Build history of the part. All positions in model axes, mm. Face numbers are marked on the shaded views. A direction names the side the tool comes from. Give positions to 0.01 mm unless a question says otherwise; leave off trailing zeros. Order: outer loops, then holes, each group sorted by start corner. A loop starts at its lowest first (then second) coordinate and runs counter-clockwise, first axis right, second up. Notation, with made-up numbers: (53, -28) - (76, -28) arc R14 cw to (76, -2) - close; hole circle Ø11 at (23.25, -38.75). An arc over 180 degrees is marked (long way). Use a Markdown table: item, result. Add a question column.
(1) Flat gauge pins, fed straight in: pin 1 (4 mm diameter, centred on x = 1.5, z = 11.5, fed in from -Y); pin 2 (6 mm diameter, centred on y = -23.5, z = 13.5, fed in from +X); pin 3 (2.5 mm diameter, centred on x = 68, z = 13, fed in from -Y). Where does each tip first touch, or does it go through?
(2) Slice it at B-B (z = 7.75). Write the cut outline in (x, y), then the cut area to 3 significant figures.
(3) Slice it at A-A (y = -28.5). Write the cut outline in (x, z), then the cut area to 3 significant figures.
(4) Wall check: line 1 (X direction, y = -19.5, z = 16.5); line 2 (X direction, y = -33, z = 14.5); line 3 (Y direction, x = 62, z = 2). Give the ranges that are in metal, low to high.
(5) Which spindle directions (+Z, -Z, +X, -X, +Y, -Y) get a long thin tool onto all of the face, cutting with end or side? Do the marked faces 1, 2 and 3. Say none if no direction does.
(6) Mould opens along X. For the marked faces 4, 5, 6 and 7 say: +X half, -X half, draft (parallel to the pull), parting line (faces both ways), or undercut.
(7) Slice it at C-C (x = 68). Write the cut outline in (y, z).
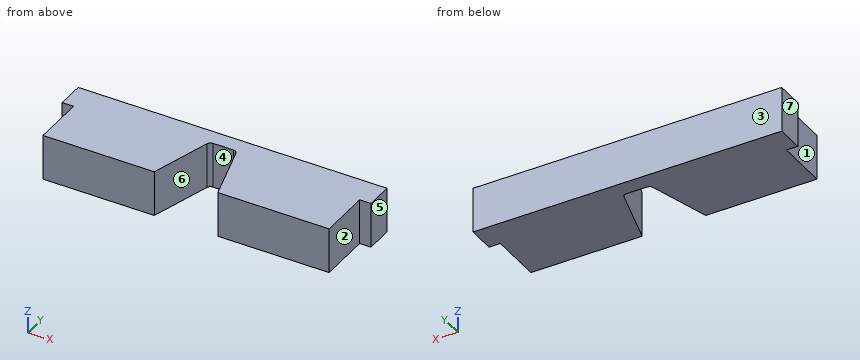
from build123d import *

# Parameters (mm, degrees)
F0_W     = 136
F0_H     = 35
F1_DEPTH = 20
F2_W     = 5
F2_H     = 23
F3_DEPTH = 25
F4_R     = 2


with BuildPart() as f1:
    # F0 (on Top) → F1 (new body)
    with BuildSketch(Plane.XY):
        with Locations((68, -17.5)):
            Rectangle(F0_W, F0_H)
    extrude(amount=F1_DEPTH)

    # F2 (on face) → F3 (cut)
    with BuildSketch(Plane.XY.offset(20)):
        Polygon((68, -7), (62, -7), (54, -35), (82, -35), (74, -7), align=None)
        with Locations((133.5, -23.5)):
            Rectangle(F2_W, F2_H)
        with Locations((2.5, -23.5)):
            Rectangle(F2_W, F2_H)
    extrude(amount=-F3_DEPTH, mode=Mode.SUBTRACT)

    # F4
    f4_edges = [f1.edges().sort_by_distance(p)[0] for p in [
        (62, -7, 10),
        (74, -7, 10),
    ]]
    fillet(f4_edges, radius=F4_R)


solid = f1.part
Solution:
| question | item | result |
|---|---|---|
| 1 | pin 1 | y = -12 |
| 1 | pin 2 | x = 131 |
| 1 | pin 3 | y = -7 |
| 2 | outline | (0, -12) - (5, -12) - (5, -35) - (54, -35) - (61.59, -8.45) arc R2 cw to (63.51, -7) - (72.49, -7) arc R2 cw to (74.41, -8.45) - (82, -35) - (131, -35) - (131, -12) - (136, -12) - (136, 0) - (0, 0) - close |
| 2 | area | 3,970 mm2 |
| 3 | outline | (5, 0) - (55.86, 0) - (55.86, 20) - (5, 20) - close; (80.14, 0) - (131, 0) - (131, 20) - (80.14, 20) - close |
| 3 | area | 2,030 mm2 |
| 4 | line 1 | 5 to 58.43, 77.57 to 131 |
| 4 | line 2 | 5 to 54.57, 81.43 to 131 |
| 4 | line 3 | -7.69 to 0 |
| 5 | face 1 | +Z, -Z, -X, -Y |
| 5 | face 2 | +Z, -Z, +X, -Y |
| 5 | face 3 | +Z, -Z, +X, -X, +Y |
| 6 | face 4 | undercut |
| 6 | face 5 | +X half |
| 6 | face 6 | undercut |
| 6 | face 7 | -X half |
| 7 | outline | (-7, 0) - (0, 0) - (0, 20) - (-7, 20) - close |
